CAD build for the part. Positions are in the model's coordinates, mm. A direction names the side the tool comes from. Coordinates: 2 decimals unless noted, no trailing zeros. Order: outer loops, then holes, each group sorted by start corner. A loop starts at its lowest first (then second) coordinate and runs counter-clockwise, first axis right, second up. Notation, with made-up numbers: (-4, -18) -> (13, -18) arc R28 cw to (13, 15) -> close; hole circle Ø1 at (-3, -35.75). An arc over 180 degrees is marked (long way). Use one line per item in the form item = value. Start each with the question number.
from build123d import *

# Parameters (mm, degrees)
F0_R     = 4
F1_DEPTH = 6
F2_DEPTH = 6
F0_W     = 12.7
F0_H     = 6
F3_DEPTH = 25


with BuildPart() as f1:
    # F0 (on Top) → F1 (new body)
    with BuildSketch(Plane.XY):
        with BuildLine():
            ThreePointArc((-14.991796, -6), (-13.292449, -3.211399), (-12.7, 0))
            ThreePointArc((-12.7, 0), (-13.292449, 3.211399), (-14.991796, 6))
            ThreePointArc((-14.991796, 6), (-30.7, 0), (-14.991796, -6))
        make_face()
        with Locations((-21.7, 0)):
            Circle(F0_R, mode=Mode.SUBTRACT)
    extrude(amount=F1_DEPTH)

    # F0 (on Top) → F2 (join)
    with BuildSketch(Plane.XY):
        with BuildLine():
            Line((-12.7, -6), (-12.7, 0))
            ThreePointArc((-12.7, 0), (-13.292449, -3.211399), (-14.991796, -6))
            Line((-14.991796, -6), (-12.7, -6))
        make_face()
        with BuildLine():
            ThreePointArc((-14.991796, 6), (-13.292449, 3.211399), (-12.7, 0))
            Line((-12.7, 0), (-12.7, 6))
            Line((-12.7, 6), (-14.991796, 6))
        make_face()
    extrude(amount=F2_DEPTH)

    # F0 (on Top) → F3 (join)
    with BuildSketch(Plane.XY):
        with Locations((-6.35, -3)):
            Rectangle(F0_W, F0_H)
        with Locations((-6.35, 3)):
            Rectangle(F0_W, F0_H)
    extrude(amount=F3_DEPTH)


solid = f1.part
1) Drop flat-ended pins along their axis: P1, Ø2, axis at x = -5.5, z = 17.5, coming from the +Y side; P2, Ø2, axis at x = -19.5, z = 6.5, coming from the -Y side; P3, Ø5.5, axis at x = -25.5, y = 4, coming from the +Z side; P4, Ø2, axis at x = -22, y = -1, coming from the -Z side. Give the stop position or say it passes through.
2) 3-axis set-ups, long thin cutter, end or side, ignore diameter. For faces 4 (the face through (-8, -6, 12)), 5 (the face through (-30.695, 0.304, 2.958)), 6 (the face through (-12.7, 0, 15)), 7 (the face through (-8, 6, 12)): which of +Z, -Z, +X, -X, +Y, -Y reach the whole face in a straight line?
3) Probe L1, parallel to Y at x = -21.7, z = 2.25; L2, parallel to Y at x = -12, z = 12; L3, parallel to Z at x = -29, y = -0.5. List the from-to ranges inside material, lowest first.
4) Two-plate mould, pull along X, no slides. Class faces 1 (the face through (-18, -2, 6)), 2 (the face through (0, 0, 12)), 3 (the face through (-18.005, -1.532, 2.958)): released by +X, released by -X, zero draft, split by the parting line, or undercut.
5) Cut at B-B on x = -21.7. Give the cut face in (y, z), then the cut area to 3 significant figures.
6) Cut at A-A on y = 0. Give the cut face in (x, z).
7) Cut at C-C on x = -9.5. Give the cut face in (y, z), then the cut area to 3 significant figures.
8) Cut at D-D on z = 14. Give the cut face in (x, y).
Values follow:
q1.P1 = 6
q1.P2 = -8.9
q1.P3 = 6
q1.P4 = through
q2.face_4 = +Z, -Z, +X, -Y
q2.face_5 = +Z, -Z
q2.face_6 = +Z, -X, +Y, -Y
q2.face_7 = +Z, -Z, +X, +Y
q3.L1 = -9 to -4, 4 to 9
q3.L2 = -6 to 6
q3.L3 = 0 to 6
q4.face_1 = zero draft
q4.face_2 = released by +X
q4.face_3 = undercut
q5.outline = (-9, 0) -> (-4, 0) -> (-4, 6) -> (-9, 6) -> close; (4, 0) -> (9, 0) -> (9, 6) -> (4, 6) -> close
q5.area = 60.0 mm^2
q6.outline = (-30.7, 0) -> (-25.7, 0) -> (-25.7, 6) -> (-30.7, 6) -> close; (-17.7, 0) -> (0, 0) -> (0, 25) -> (-12.7, 25) -> (-12.7, 6) -> (-17.7, 6) -> close
q7.outline = (-6, 0) -> (6, 0) -> (6, 25) -> (-6, 25) -> close
q7.area = 300 mm^2
q8.outline = (-12.7, -6) -> (0, -6) -> (0, 6) -> (-12.7, 6) -> close
